from build123d import *

# Parameters (mm, degrees)
ESQUISSE1_W             = 15
ESQUISSE1_H             = 50
BOSS_EXTRU_1_DEPTH      = 30
ESQUISSE2_W             = 3.6
ESQUISSE2_H             = 50
ENL_V_MAT_EXTRU_1_DEPTH = 24.3
BOSS_EXTRU_2_DEPTH      = 50
ESQUISSE5_W             = 3.6
ESQUISSE5_H             = 24.3
ENL_V_MAT_EXTRU_2_DEPTH = 2


with BuildPart() as part:
    # Esquisse1 → Boss.-Extru.1 (new body)
    with BuildSketch(Plane.XY):
        with Locations((7.5, -25)):
            Rectangle(ESQUISSE1_W, ESQUISSE1_H)
    extrude(amount=BOSS_EXTRU_1_DEPTH)

    # Esquisse2 → Enlèv. mat.-Extru.1 (cut)
    with BuildSketch(Plane.XY.offset(30)):
        with Locations((7.5, -25)):
            Rectangle(ESQUISSE2_W, ESQUISSE2_H)
    extrude(amount=-ENL_V_MAT_EXTRU_1_DEPTH, mode=Mode.SUBTRACT)

    # Esquisse4 → Boss.-Extru.2 (add)
    with BuildSketch(Plane(origin=(15, 0, 0), x_dir=(0, 0, -1), z_dir=(1, 0, 0))):
        Polygon((0, -50), (0, -20), (-15, -20), (-15, -50), (-9.3, -50), (-9.3, -25.7), (-5.7, -25.7), (-5.7, -50), align=None)
    extrude(amount=BOSS_EXTRU_2_DEPTH)

    # Esquisse5 → Enlèv. mat.-Extru.2 (cut)
    with BuildSketch(Plane(origin=(15, 0, 0), x_dir=(0, 0, -1), z_dir=(1, 0, 0))):
        with Locations((-7.5, -37.85)):
            Rectangle(ESQUISSE5_W, ESQUISSE5_H)
    extrude(amount=-ENL_V_MAT_EXTRU_2_DEPTH, mode=Mode.SUBTRACT)


solid = part.part
Model file for the job. Use its own axes, mm. A direction names the side the tool comes from. Give positions to 0.01 mm unless a question says otherwise; leave off trailing zeros. Order: outer loops, then holes, each group sorted by start corner. A loop starts at its lowest first (then second) coordinate and runs counter-clockwise, first axis right, second up. Notation, with made-up numbers: M -10.5,0.5 L -3.5,0.5 A10 ccw -3.5,9.5 Z; hole C -12.75,7 d9. An arc over 180 degrees is marked long. Put each result on its own line as item: value. Start each with the question number.
(1) Band-saw the part on B-B on x = 45.5. Give the cut face in (y, z).
(2) Band-saw the part on D-D on z = 4.5. Give the cut face in (x, y).
(3) Pull direction X, two halves, no side cores. Call faces 1 (the face through (7, -25, 5.7)), 2 (the face through (0, -25, 15)), 3 (the face through (25, -50, 12)), 4 (the face through (5.7, -25, 18)): released by +X, released by -X, zero draft, split by the parting line, or undercut.
(4) Band-saw the part on A-A on z = 11.25. Give the cut face in (x, y), then the cut area to 3 significant figures.
(5) Pin check, flat tips, straight feed: pin 1 Ø16.5 at (x, z) = (27.5, 9.5) entering from +Y; pin 2 Ø3 at (y, z) = (-44, 7.5) entering from +X; pin 3 Ø6 at (x, y) = (46, -20) entering from +Z. Stop position of each tip, or through.
(6) Tool access for faces 5 (the face through (40, -35, 15)), 6 (the face through (9.3, -25, 18)), 7 (the face through (39, -38, 9.3)), 8 (the face through (40, -20, 7)): list every direction of +Z, -Z, +X, -X, +Y, -Y with a clear straight run to the whole face (end or side of a thin tool).
(7) Band-saw the part on C-C on y = -25. Give the cut face in (x, z).
(8) Drill centre lines: L1, parallel to X at y = -18, z = 26.75; L2, parallel to X at y = -38, z = 7.25. Where is each one in solid material? Low to high. Write a range as [from, to].
Results below:
1. outline: M -50,0 L -20,0 L -20,15 L -50,15 L -50,9.3 L -25.7,9.3 L -25.7,5.7 L -50,5.7 Z
2. outline: M 0,-50 L 65,-50 L 65,-20 L 15,-20 L 15,0 L 0,0 Z
3. face 1: undercut
3. face 2: released by -X
3. face 3: zero draft
3. face 4: undercut
4. outline: M 0,-50 L 5.7,-50 L 5.7,0 L 0,0 Z; M 9.3,-50 L 65,-50 L 65,-20 L 15,-20 L 15,0 L 9.3,0 Z
4. area: 2,070 mm2
5. pin 1: stops at y = -20
5. pin 2: stops at x = 13
5. pin 3: stops at z = 15
6. face 5: +Z, +X, +Y, -Y
6. face 6: +Z, +Y, -Y
6. face 7: +X, -Y
6. face 8: +Z, -Z, +X, +Y
7. outline: M 0,0 L 65,0 L 65,15 L 15,15 L 15,30 L 9.3,30 L 9.3,5.7 L 5.7,5.7 L 5.7,30 L 0,30 Z
8. L1: x = [0, 5.7], [9.3, 15]
8. L2: x = [0, 5.7], [9.3, 13]
